Read the model definition and answer for the solid it produces. Units are mm, in the model's axes. A direction names the side the tool comes from. Coordinates: 2 decimals unless noted, no trailing zeros. Order: outer loops, then holes, each group sorted by start corner. A loop starts at its lowest first (then second) coordinate and runs counter-clockwise, first axis right, second up.
```python
from build123d import *

# Parameters (mm, degrees)
F0_R      = 25.4
F0_R_2    = 7.9375
F1_DEPTH  = 57.912
F2_SIZE2  = 11.8776606661
F2_SIZE   = 55.88
F3_R      = 34.7599
F3_R_2    = 13.5223393339
F3_R_3    = 7.9375
F4_DEPTH  = 12.192
F6_R      = 32.2199
F6_R_2    = 8.4234043
F7_DEPTH  = 2.54
F8_R      = 34.7754798106
F8_R_2    = 32.2199
F8_R_3    = 8.4234043
F9_DEPTH  = 3.81
F10_R     = 32.2199
F10_R_2   = 8.4234043
F11_DEPTH = 2.54
F13_R     = 34.7599
F13_R_2   = 32.2199
F12_R     = 32.2199
F12_R_2   = 8.4234043
F14_DEPTH = 6.858
F15_SIZE2 = 14.6646968374
F15_SIZE  = 25.4


# Not quite as in the source:
# - a fillet or chamfer that OpenCascade refuses, or shapes differently, is made with other operations: its cross-section is extruded or revolved along the edge and cut away or added


with BuildPart() as f1:
    # F0 (on Front) → F1 (new body)
    with BuildSketch(Plane.XZ):
        Circle(F0_R)
        Circle(F0_R_2, mode=Mode.SUBTRACT)
    extrude(amount=F1_DEPTH)

    # F2
    f2_edges = [f1.edges().sort_by_distance(p)[0] for p in [
        (-25.4, 0, 0),
    ]]
    f2_side = f1.faces().sort_by_distance((-25.4, -28.956, 0))[0]
    chamfer(f2_edges, length=F2_SIZE, length2=F2_SIZE2, reference=f2_side)

    # F3 (on face) → F4 (join)
    with BuildSketch(Plane(origin=(0, 0, 0), x_dir=(-1, 0, 0), z_dir=(0, 1, 0))):
        Circle(F3_R)
        Circle(F3_R_2, mode=Mode.SUBTRACT)
        Circle(F3_R_2)
        Circle(F3_R_3, mode=Mode.SUBTRACT)
    extrude(amount=F4_DEPTH)

    # F5: chamfer of 72.39 x 15.3869694993 on 1 edges, made by hand

    # F5_s1 → F5_t2 (revolve, cut)
    with BuildSketch(Plane.XY):
        Polygon((23.3244694993, -57.912), (7.9375, 14.478), (7.9375, -57.912), align=None)
    revolve(axis=Axis((0, -57.912, 0), (0, -1, 0)), mode=Mode.SUBTRACT)

    # F6 (on face) → F7 (join)
    with BuildSketch(Plane(origin=(0, 12.192, 0), x_dir=(-1, 0, 0), z_dir=(0, 1, 0))):
        Circle(F6_R)
        Circle(F6_R_2, mode=Mode.SUBTRACT)
    extrude(amount=F7_DEPTH)

    # F8 (on face) → F9 (join)
    with BuildSketch(Plane(origin=(0, 14.732, 0), x_dir=(-1, 0, 0), z_dir=(0, 1, 0))):
        Circle(F8_R)
        Circle(F8_R_2, mode=Mode.SUBTRACT)
        Circle(F8_R_2)
        Circle(F8_R_3, mode=Mode.SUBTRACT)
    extrude(amount=F9_DEPTH)

    # F10 (on face) → F11 (join)
    with BuildSketch(Plane(origin=(0, 18.542, 0), x_dir=(-1, 0, 0), z_dir=(0, 1, 0))):
        Circle(F10_R)
        Circle(F10_R_2, mode=Mode.SUBTRACT)
    extrude(amount=F11_DEPTH)

    # F13 (on face) + F12 (on face) → F14 (join)
    with BuildSketch(Plane(origin=(0, 21.082, 0), x_dir=(-1, 0, 0), z_dir=(0, 1, 0))):
        Circle(F13_R)
        Circle(F13_R_2, mode=Mode.SUBTRACT)
    with BuildSketch(Plane(origin=(0, 21.082, 0), x_dir=(-1, 0, 0), z_dir=(0, 1, 0))):
        Circle(F12_R)
        Circle(F12_R_2, mode=Mode.SUBTRACT)
    extrude(amount=F14_DEPTH)

    # F15
    f15_edges = [f1.edges().sort_by_distance(p)[0] for p in [
        (8.423404, 27.94, 0),
    ]]
    f15_side = f1.faces().sort_by_distance((33.776742, 27.94, 0))[0]
    chamfer(f15_edges, length=F15_SIZE, length2=F15_SIZE2, reference=f15_side)


solid = f1.part
```
1) Flat-ended cylindrical pins translate along their axes: pin 1 Ø4 at (x, z) = (0.5, 6.5) entering from +Y; pin 2 Ø8 at (y, z) = (-12, 7) entering from -X; pin 3 Ø10 at (x, z) = (7, -0.5) entering from +Y. Find the tip coordinate at first contact, or state that the pin passes through.
A:
pin 1: stops at y = 13.33
pin 2: stops at x = -16.15
pin 3: stops at y = 15.35
2) Straight lines are drawn through the part: line 1 (Z direction, x = 0, y = 12.95); line 2 (X direction, y = -53.5, z = -15); line 3 (Z direction, x = -14, y = -47.5). For each, find the intervals that lie inside material, in ascending order.
A:
line 1: z = -32.22 to -8.42, 8.42 to 32.22
line 2: x = -19.87 to -16.62, 16.62 to 19.87
line 3: z = -19.02 to -15.8, 15.8 to 19.02
3) A cutting plane is placed at D-D, the plane y = -21.5. Determine the outline of the cut face in (x, z).
A:
outline: circle Ø36.18 at (0, 0); hole circle Ø31.17 at (0, 0)
4) Determine the mould class of faces 4 (the conical face through (2.09, 13.99, -9.43)), 5 (the cylindrical face through (27.597, 16.61, -21.16)), 6 (the flat face through (11, -57.912, -21)) for opening direction Z: pulls with the +Z half, pulls with the -Z half, needs draft (parallel to the pull), parting line crosses it, or undercut.
A:
face 4: undercut
face 5: parting line crosses it
face 6: needs draft
5) A cutting plane is placed at C-C, the plane y = 10.5. Determine the outline of the cut face in (x, z).
A:
outline: circle Ø69.52 at (0, 0); hole circle Ø17.57 at (0, 0)
6) Which of the six approach directions +Z, -Z, +X, -X, +Y, -Y give full straight-line access (tool end or side, diameter ignored) to faces 1 (the cylindrical face through (-5.506, -56.882, -24.796)), 2 (the flat face through (-7.6, 27.94, -33.3)), 3 (the cylindrical face through (25.569, 13.444, -19.605))?
A:
face 1: -Y
face 2: +Z, -Z, +X, -X, +Y
face 3: none
